Read the model definition and answer for the solid it produces. Units are mm, in the model's axes. Face numbers are marked on the shaded views. A direction names the side the tool comes from. Coordinates: 2 decimals unless noted, no trailing zeros. Loops run counter-clockwise (first coordinate to the right, second up) from the corner with the lowest first, then second, coordinate; pieces in that order, holes last. Notation, with made-up numbers: (-22.75, 80) - (31.25, 80) arc R12 cw to (31.25, 87) - close; hole circle Ø10 at (31, 30). An arc over 180 degrees is marked (long way). Use one line per item in the form item = value. Start each with the question number.
1) A cutting plane is placed at C-C (x = -31). Give the vertices of the cut face in (y, z).
2) A cutting plane is placed at A-A (y = 18.5). Give the vertices of the cut face in (x, z).
3) A cutting plane is placed at B-B (z = -2.5). Give the vertices of the cut face in (x, y).
4) The mould has two halves that part along X. Classify the marked faces 3, 4, 5 and 6: released by +X, released by -X, zero draft, split by the parting line, or undercut.
5) Consider line 1 (X direction, y = 25, z = -54); line 2 (X direction, y = 5.5, z = -44.5). Determine where each line is inside the solid, lowest interval first.
6) A cutting plane is placed at D-D (y = 36.5). Give the vertices of the cut face in (x, z).
7) Which of the six approach directions +Z, -Z, +X, -X, +Y, -Y give full straight-line access (tool end or side, diameter ignored) to the marked faces 1 and 2?
8) Each of these flat-tipped pins is pushed along its axis until it touches: P1, Ø1.8, axis at x = 33, z = 43.5, coming from the +Y side; P2, Ø1.8, axis at x = -25.5, z = 42.5, coming from the +Y side; P3, Ø2, axis at y = 11, z = 21, coming from the +X side. Where does it stop, or does it pass through?
from build123d import *

# Parameters (mm, degrees)
SKETCH1_W           = 120
SKETCH1_H           = 120
BOSS_EXTRUDE1_DEPTH = 2
SKETCH3_R           = 3
SKETCH3_R_2         = 2.15
BOSS_EXTRUDE2_DEPTH = 6
SKETCH4_W           = 120
SKETCH4_H           = 120
SKETCH4_W_2         = 118
SKETCH4_H_2         = 118
BOSS_EXTRUDE3_DEPTH = 40
SKETCH5_W           = 15.299999553
SKETCH5_H           = 16.42
SKETCH5_W_2         = 32.63620328
SKETCH5_H_2         = 14.399997005
SKETCH5_W_3         = 11.5
SKETCH5_H_3         = 5.5
CUT_EXTRUDE1_DEPTH  = 1


with BuildPart() as part:
    # Sketch1 → Boss-Extrude1 (new body)
    with BuildSketch(Plane(origin=(0, 0, 0), x_dir=(1, 0, 0), z_dir=(0, 1, 0))):
        Rectangle(SKETCH1_W, SKETCH1_H)
    extrude(amount=BOSS_EXTRUDE1_DEPTH)

    # Sketch3 → Boss-Extrude2 (add)
    with BuildSketch(Plane(origin=(0, 2, 0), x_dir=(1, 0, 0), z_dir=(0, 1, 0))):
        with Locations((-24.500233826, 46.14332907)):
            Circle(SKETCH3_R)
        with Locations((-24.500233826, 46.14332907)):
            Circle(SKETCH3_R_2, mode=Mode.SUBTRACT)
        with Locations((33.499766618, 46.136550123)):
            Circle(SKETCH3_R)
        with Locations((33.499766618, 46.136550123)):
            Circle(SKETCH3_R_2, mode=Mode.SUBTRACT)
        with Locations((33.801832122, -42.455500627)):
            Circle(SKETCH3_R)
        with Locations((33.801832122, -42.455500627)):
            Circle(SKETCH3_R_2, mode=Mode.SUBTRACT)
        with Locations((-24.541068319, -42.448681603)):
            Circle(SKETCH3_R)
        with Locations((-24.541068319, -42.448681603)):
            Circle(SKETCH3_R_2, mode=Mode.SUBTRACT)
    extrude(amount=BOSS_EXTRUDE2_DEPTH)

    # Sketch4 → Boss-Extrude3 (add)
    with BuildSketch(Plane(origin=(0, 2, 0), x_dir=(1, 0, 0), z_dir=(0, 1, 0))):
        Rectangle(SKETCH4_W, SKETCH4_H)
        Rectangle(SKETCH4_W_2, SKETCH4_H_2, mode=Mode.SUBTRACT)
    extrude(amount=BOSS_EXTRUDE3_DEPTH)

    # Sketch5 → Cut-Extrude1 (cut)
    with BuildSketch(Plane(origin=(60, 0, 0), x_dir=(0, 0, -1), z_dir=(1, 0, 0))):
        with Locations((-22.123446946, 16.599997028)):
            Rectangle(SKETCH5_W, SKETCH5_H)
        with BuildLine():
            Line((-6.960880715, 24.719998619), (-7.078005207, 24.349104393))
            Line((-7.078005207, 24.349104393), (-7.938323111, 23.560479642))
            add(Edge.make_bspline(
                [(-7.938323111, 23.560479642), (-8.008708428, 23.495959767), (-8.135677464, 23.353602564), (-8.283483399, 23.096453844), (-8.373165531, 22.813736363), (-8.392308628, 22.623946344), (-8.392308628, 22.528463847)],
                knots=[0, 0, 0, 0, 0.25, 0.5, 0.75, 1, 1, 1, 1], degree=3))
            Line((-8.392308628, 22.528463847), (-8.392308628, 13.068365563))
            add(Edge.make_bspline(
                [(-8.392308628, 13.068365563), (-8.392308628, 12.972883067), (-8.373165531, 12.783093048), (-8.283483399, 12.500375567), (-8.135677464, 12.243226847), (-8.008708428, 12.100869643), (-7.938323111, 12.036349768)],
                knots=[0, 0, 0, 0, 0.25, 0.5, 0.75, 1, 1, 1, 1], degree=3))
            Line((-7.938323111, 12.036349768), (-7.078005207, 11.247725017))
            Line((-7.078005207, 11.247725017), (-6.960880715, 10.876830791))
            add(Edge.make_bspline(
                [(-6.960880715, 10.876830791), (-6.917752001, 10.740256529), (-6.792916696, 10.483611985), (-6.46908795, 10.147865428), (-6.051410861, 9.940171767), (-5.769087247, 9.898414705), (-5.625864989, 9.898414705)],
                knots=[0, 0, 0, 0, 0.25, 0.5, 0.75, 1, 1, 1, 1], degree=3))
            Line((-5.625864989, 9.898414705), (-3.442308658, 9.898414705))
            add(Edge.make_bspline(
                [(-3.442308658, 9.898414705), (-3.267434145, 9.898414705), (-2.925471239, 9.958566446), (-2.42155584, 10.277661886), (-2.102460404, 10.781577287), (-2.042308664, 11.123540192), (-2.042308664, 11.298414705)],
                knots=[0, 0, 0, 0, 0.25, 0.5, 0.75, 1, 1, 1, 1], degree=3))
            Line((-2.042308664, 11.298414705), (-2.042308664, 24.298414705))
            add(Edge.make_bspline(
                [(-2.042308664, 24.298414705), (-2.042308664, 24.473289219), (-2.102460404, 24.815252124), (-2.42155584, 25.319167525), (-2.925471239, 25.638262964), (-3.267434145, 25.698414705), (-3.442308658, 25.698414705)],
                knots=[0, 0, 0, 0, 0.25, 0.5, 0.75, 1, 1, 1, 1], degree=3))
            Line((-3.442308658, 25.698414705), (-5.625864989, 25.698414705))
            add(Edge.make_bspline(
                [(-5.625864989, 25.698414705), (-5.769087247, 25.698414705), (-6.051410861, 25.656657644), (-6.46908795, 25.448963983), (-6.792916696, 25.113217425), (-6.917752001, 24.856572882), (-6.960880715, 24.719998619)],
                knots=[0, 0, 0, 0, 0.25, 0.5, 0.75, 1, 1, 1, 1], degree=3))
        make_face()
        with BuildLine():
            Line((5.997249079, 24.719998619), (5.880124588, 24.349104393))
            Line((5.880124588, 24.349104393), (5.019806683, 23.560479642))
            add(Edge.make_bspline(
                [(5.019806683, 23.560479642), (4.949421366, 23.495959767), (4.82245233, 23.353602564), (4.674646395, 23.096453844), (4.584964263, 22.813736363), (4.565821167, 22.623946344), (4.565821167, 22.528463847)],
                knots=[0, 0, 0, 0, 0.25, 0.5, 0.75, 1, 1, 1, 1], degree=3))
            Line((4.565821167, 22.528463847), (4.565821167, 13.068365563))
            add(Edge.make_bspline(
                [(4.565821167, 13.068365563), (4.565821167, 12.972883067), (4.584964263, 12.783093048), (4.674646395, 12.500375567), (4.82245233, 12.243226847), (4.949421366, 12.100869643), (5.019806683, 12.036349768)],
                knots=[0, 0, 0, 0, 0.25, 0.5, 0.75, 1, 1, 1, 1], degree=3))
            Line((5.019806683, 12.036349768), (5.880124588, 11.247725017))
            Line((5.880124588, 11.247725017), (5.997249079, 10.876830791))
            add(Edge.make_bspline(
                [(5.997249079, 10.876830791), (6.040377794, 10.740256529), (6.165213099, 10.483611985), (6.489041844, 10.147865428), (6.906718933, 9.940171767), (7.189042547, 9.898414705), (7.332264805, 9.898414705)],
                knots=[0, 0, 0, 0, 0.25, 0.5, 0.75, 1, 1, 1, 1], degree=3))
            Line((7.332264805, 9.898414705), (9.515821136, 9.898414705))
            add(Edge.make_bspline(
                [(9.515821136, 9.898414705), (9.69069565, 9.898414705), (10.032658555, 9.958566446), (10.536573954, 10.277661886), (10.85566939, 10.781577287), (10.91582113, 11.123540192), (10.91582113, 11.298414705)],
                knots=[0, 0, 0, 0, 0.25, 0.5, 0.75, 1, 1, 1, 1], degree=3))
            Line((10.91582113, 11.298414705), (10.91582113, 24.298414705))
            add(Edge.make_bspline(
                [(10.91582113, 24.298414705), (10.91582113, 24.473289219), (10.85566939, 24.815252124), (10.536573954, 25.319167525), (10.032658555, 25.638262964), (9.69069565, 25.698414705), (9.515821136, 25.698414705)],
                knots=[0, 0, 0, 0, 0.25, 0.5, 0.75, 1, 1, 1, 1], degree=3))
            Line((9.515821136, 25.698414705), (7.332264805, 25.698414705))
            add(Edge.make_bspline(
                [(7.332264805, 25.698414705), (7.189042547, 25.698414705), (6.906718933, 25.656657644), (6.489041844, 25.448963983), (6.165213099, 25.113217425), (6.040377793, 24.856572882), (5.997249079, 24.719998619)],
                knots=[0, 0, 0, 0, 0.25, 0.5, 0.75, 1, 1, 1, 1], degree=3))
        make_face()
        with Locations((32.443720838, 15.498417022)):
            Rectangle(SKETCH5_W_2, SKETCH5_H_2)
        with Locations((-40.056026235, 10.14841852)):
            Rectangle(SKETCH5_W_3, SKETCH5_H_3)
    extrude(amount=-CUT_EXTRUDE1_DEPTH, mode=Mode.SUBTRACT)


solid = part.part
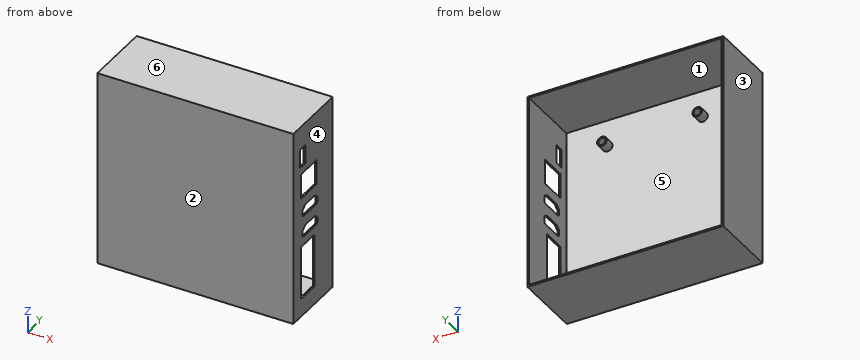
Found:
q1.outline = (0, -60) - (42, -60) - (42, -59) - (2, -59) - (2, 59) - (42, 59) - (42, 60) - (0, 60) - close
q2.outline = (-60, -60) - (60, -60) - (60, -48.76) - (59, -48.76) - (59, -59) - (-59, -59) - (-59, 59) - (59, 59) - (59, 29.77) - (60, 29.77) - (60, 60) - (-60, 60) - close; (59, -16.13) - (60, -16.13) - (60, -10.92) - (59, -10.92) - close; (59, -4.57) - (60, -4.57) - (60, 2.04) - (59, 2.04) - close; (59, 8.39) - (60, 8.39) - (60, 14.47) - (59, 14.47) - close
q3.outline = (-60, 0) - (60, 0) - (60, 42) - (59, 42) - (59, 2) - (-59, 2) - (-59, 42) - (-60, 42) - close
q4.face_3 = released by -X
q4.face_4 = released by +X
q4.face_5 = undercut
q4.face_6 = zero draft
q5.line_1 = -60 to -59, 59 to 60
q5.line_2 = -60 to -59, -27.01 to -25.89, -23.11 to -21.99, 30.99 to 32.11, 34.89 to 36.01, 59 to 60
q6.outline = (-60, -60) - (60, -60) - (60, 60) - (-60, 60) - close; hole (-59, -59) - (59, -59) - (59, 59) - (-59, 59) - close
q7.face_1 = +Y
q7.face_2 = +Z, -Z, +X, -X, -Y
q8.P1 = 8
q8.P2 = 2
q8.P3 = -59
